```python
from build123d import *

# Parameters (mm, degrees)
SKETCH1_R           = 4
BASE_FLANGE1_DEPTH  = 2
SKETCH6_R           = 4
BOSS_EXTRUDE1_DEPTH = 15
SKETCH7_R           = 3
BOSS_EXTRUDE2_DEPTH = 15
FILLET2_R           = 5


# Sheet-metal steps are written as plain solids
with BuildPart() as part:
    # Sketch1 → Base-Flange1 (new body)
    with BuildSketch(Plane(origin=(0, 0, 0), x_dir=(1, 0, 0), z_dir=(0, 1, 0))):
        with BuildLine():
            Line((8.214438599, -24.009587925), (73.867056795, -66.644896694))
            Line((73.867056795, -66.644896694), (80.294932891, -58.984452263))
            Line((80.294932891, -58.984452263), (24.288495613, -11.989471399))
            ThreePointArc((24.288495613, -11.989471399), (13.747688519, 1.747575857), (10, 18.652306326))
            Line((10, 18.652306326), (10, 97.819006808))
            Line((10, 97.819006808), (-10, 97.819006808))
            Line((-10, 97.819006808), (-10, 9.537234793))
            ThreePointArc((-10, 9.537234793), (-5.152684506, -9.549115617), (8.214438599, -24.009587925))
        make_face()
        with Locations(Location((24.288495613, -25.043544292, 0), (0, 0, 270))):
            Circle(SKETCH1_R, mode=Mode.SUBTRACT)
        with Locations(Location((57.054577384, -47.986601746, 0), (0, 0, 270))):
            Circle(SKETCH1_R, mode=Mode.SUBTRACT)
    extrude(amount=-BASE_FLANGE1_DEPTH)

    # Sketch6 → Boss-Extrude1 (add)
    with BuildSketch(Plane.XZ.offset(2)):
        Polygon((8.214438599, 24.009587925), (73.867056795, 66.644896694), (80.294932891, 58.984452263), (24.288495613, 11.989471399), align=None)
        with Locations(Location((24.288495613, 25.043544292, 0), (0, 0, 90))):
            Circle(SKETCH6_R, mode=Mode.SUBTRACT)
        with Locations(Location((57.054577384, 47.986601746, 0), (0, 0, 90))):
            Circle(SKETCH6_R, mode=Mode.SUBTRACT)
    extrude(amount=BOSS_EXTRUDE1_DEPTH)

    # Sketch7 → Boss-Extrude2 (add)
    with BuildSketch(Plane(origin=(0, 0, 0), x_dir=(1, 0, 0), z_dir=(0, 1, 0))):
        with Locations(Location((0, 87, 0), (0, 0, 90))):
            Circle(SKETCH7_R)
    extrude(amount=BOSS_EXTRUDE2_DEPTH)

    # Fillet2
    fillet2_edges = [part.edges().sort_by_distance(p)[0] for p in [
        (73.867056795, -8.5, 66.644896694),
        (-10, -1, -97.819006808),
        (10, -1, -97.819006808),
        (80.294932891, -8.5, 58.984452263),
    ]]
    fillet(fillet2_edges, radius=FILLET2_R)


solid = part.part
```
Geometry check sheet. Reference: the model listing, model coordinates, mm. A direction names the side the tool comes from. Coordinates: 2 decimals unless noted, no trailing zeros. Write each loop counter-clockwise with the first axis right and the second up, starting at its lowest first coordinate (ties: lowest second). Pieces come first, ordered by that corner, then holes. Notation, with made-up numbers: (-35.75, 36.25) -> (-4.75, 36.25) arc R7 cw to (-4.75, 49.25) -> close; hole circle Ø3 at (33.25, 78.25). An arc over 180 degrees is marked (long way). Use CSV: the item, a comma, the result in double quotes. Start each with the question number.
Item 1: Cross-section at D-D, the plane y = 11. Record the cut outline in (x, z).
Item 2: Set-up check for faces 1 (the flat face through (16.36, -9.4, 17.92)), 2 (the cylindrical face through (73.569, -8.381, 64.995)), 3 (the cylindrical face through (0, 7, -84)): record each of +Z, -Z, +X, -X, +Y, -Y from which the full face is reachable in a straight line by a thin tool's end or side.
Item 3: Cross-section at A-A, the plane z = -87. Record the cut outline in (x, y), plus the area to 3 significant figures.
Item 4: Thickness scan on line 1 (Y direction, x = -5.5, z = -57); line 2 (X direction, y = -10.5, z = 26); line 3 (Z direction, x = 23, y = -12.5). Record the ranges inside material, lowest first.
Item 5: Cross-section at B-B, the plane y = -13.5. Record the cut outline in (x, z), plus the area to 3 significant figures.
Item 6: Cross-section at C-C, the plane x = 0. Record the cut outline in (y, z).
Item 7: Depth check by flat-ended pin: pin 1 Ø6 at (x, y) = (13, -7.5) entering from +Z; pin 2 Ø1 at (y, z) = (-1.5, -47) entering from +X; pin 3 Ø13 at (x, z) = (57.05, 47.99) entering from +Y. Enter the tip coordinate at first touch or a pass-through.
Answers:
1,outline,"circle Ø6 at (0, -87)"
2,face 1,"-Z, -X, -Y"
2,face 2,"+Z, +Y, -Y"
2,face 3,"+Y"
3,outline,"(-10, -2) -> (10, -2) -> (10, 0) -> (3, 0) -> (3, 15) -> (-3, 15) -> (-3, 0) -> (-10, 0) -> close"
3,area,"130 mm^2"
4,line 1,"-2 to 0"
4,line 2,"11.28 to 20.4, 28.17 to 40.99"
4,line 3,"12.95 to 21.26, 28.83 to 33.61"
5,outline,"(8.21, 24.01) -> (24.29, 11.99) -> (76.46, 55.77) arc R5 ccw to (77.08, 62.81) -> (76.71, 63.26) arc R5 ccw to (70.16, 64.24) -> close; hole circle Ø8 at (24.29, 25.04); hole circle Ø8 at (57.05, 47.99)"
5,area,"993 mm^2"
6,outline,"(-2, -97.82) -> (0, -97.82) -> (0, -90) -> (15, -90) -> (15, -84) -> (0, -84) -> (0, 16.92) -> (-2, 16.92) -> close"
7,pin 1,"z = 29.07"
7,pin 2,"x = 10"
7,pin 3,"y = 0"
